Autodesk Inventor part; units mm, degrees
ref_plane "YZ Plane" through (0, 0, 0) normal (1, 0, 0) x (0, 1, 0)
ref_plane "XZ Plane" through (0, 0, 0) normal (0, 1, 0) x (-1, 0, 0)
ref_plane "XY Plane" through (0, 0, 0) normal (0, 0, 1) x (1, 0, 0)
sketch "Body" plane through (0, 0, 0) normal (0, 0, 1) x (1, 0, 0)
  line L0 (-13.716, -23.495) -> (13.716, -23.495)
  line L1 (13.716, -23.495) -> (13.716, 23.495)
  line L2 (13.716, 23.495) -> (-13.716, 23.495)
  line L3 (-13.716, 23.495) -> (-13.716, -23.495)
  line L4 (-13.716, -23.495) -> (13.716, 23.495) construction
  line L5 (13.716, -23.495) -> (-13.716, 23.495) construction
  point P0 (0, 0)
  dimension "d0" = 27.432
  dimension "d1" = 46.99
extrude "BodyFeature" add sketch "Body" along normal blind 22.606
chamfer "OutsideChamfersFeature" distance 6 angle 45 2 edges at (13.716, 23.495, 11.303) (-13.716, 23.495, 11.303)
sketch "Mount" plane through (0, 0, 22.606) normal (0, 0, 1) x (1, 0, 0)
  line L0 (-24.5, -29.5) -> (24.5, -29.5) construction
  line L1 (24.5, -29.5) -> (24.5, 29.5) construction
  line L2 (24.5, 29.5) -> (-24.5, 29.5) construction
  line L3 (-24.5, 29.5) -> (-24.5, -29.5) construction
  line L4 (-24.5, -29.5) -> (24.5, 29.5) construction
  line L5 (24.5, -29.5) -> (-24.5, 29.5) construction
  line L6 (-13.5, 29.5) -> (13.5, 29.5)
  line L7 (-13.5, 29.5) -> (-24.5, 0)
  line L8 (13.5, 29.5) -> (24.5, 0)
  line L9 (-33.6, 0) -> (33.6, 0) construction
  line L10 (-13.5, -29.5) -> (13.5, -29.5)
  line L11 (-13.5, -29.5) -> (-24.5, 0)
  line L12 (13.5, -29.5) -> (24.5, 0)
  point P0 (0, 0)
  point P1 (0, 29.5)
  dimension "d7" = 59
  dimension "d8" = 49
  dimension "d9" = 27
extrude "MountFeature" add sketch "Mount" along normal blind 2.32
fillet "MountFilletsFeature" radius 1 6 edges at (-13.5, 29.5, 23.766) (13.5, 29.5, 23.766) (-24.5, 0, 23.766) (24.5, 0, 23.766) (13.5, -29.5, 23.766) (-13.5, -29.5, 23.766)
sketch "MountHoles" plane through (0, 0, 24.926) normal (0, 0, 1) x (1, 0, 0)
  line L0 (-34.3, 0) -> (34.3, 0) construction
  circle A0 centre (-20, 0) radius 1.75
  line L1 (0, -41.3) -> (0, 41.3) construction
  circle A1 centre (20, 0) radius 1.75
  point P0 (0, 0)
  dimension "d13" = 3.5
  dimension "d14" = 40
extrude "MountHolesFeature" cut sketch "MountHoles" against normal blind 3.5
sketch "FrontPanel" plane through (0, 0, 24.926) normal (0, 0, 1) x (1, 0, 0)
  line L0 (-14.15, -27.7568) -> (14.15, -27.7568)
  line L1 (14.15, -27.7568) -> (14.15, 27.7568)
  line L2 (14.15, 27.7568) -> (-14.15, 27.7568)
  line L3 (-14.15, 27.7568) -> (-14.15, -27.7568)
  line L4 (-14.15, -27.7568) -> (14.15, 27.7568) construction
  line L5 (14.15, -27.7568) -> (-14.15, 27.7568) construction
  line L6 (24.3697, 0.3494) -> (13.7426, 28.8494) construction
  point P0 (0, 0)
  dimension "d17" = 28.3
extrude "FrontPanelFeature" add sketch "FrontPanel" along normal blind 0.5
fillet "FrontPanelFilletsFeature" radius 1 4 edges at (-14.15, -27.7568, 25.176) (14.15, -27.7568, 25.176) (-14.15, 27.7568, 25.176) (14.15, 27.7568, 25.176)
sketch "PowerReceptacle" plane through (0, 0, 25.426) normal (0, 0, 1) x (1, 0, 0)
  line L0 (0, -41.3) -> (0, 41.3) construction
  line L1 (-12.3, 22) -> (12.3, 22) construction
  line L2 (12.3, 22) -> (12.3, 5.8) construction
  line L3 (12.3, 5.8) -> (-12.3, 5.8) construction
  line L4 (-12.3, 5.8) -> (-12.3, 22) construction
  line L5 (-12.3, 22) -> (12.3, 5.8) construction
  line L6 (12.3, 22) -> (-12.3, 5.8) construction
  line L7 (12.8056, 29.5) -> (-12.8056, 29.5) construction
  line L8 (-7, 22) -> (7, 22)
  line L9 (-7, 22) -> (-12.3, 17.8)
  line L10 (-12.3, 17.8) -> (-12.3, 5.8)
  line L11 (7.716, 23.495) -> (-7.716, 23.495)
  line L12 (7, 22) -> (12.3, 17.8)
  line L13 (12.3, 17.8) -> (12.3, 5.8)
  line L14 (-12.3, 5.8) -> (12.3, 5.8)
  line L15 (14.15, 26.7568) -> (14.15, -26.7568)
  point P0 (0, 0)
  point P1 (0, 13.9)
  point P2 (0, 22)
  dimension "d22" = 24.6
  dimension "d23" = 16.2
  dimension "d24" = 7.5
  dimension "d25" = 14
  dimension "d26" = 12
extrude "PowerReceptacleFeature" cut sketch "PowerReceptacle" against normal blind 18.2
sketch "Switch" plane through (0, 0, 25.426) normal (0, 0, 1) x (1, 0, 0)
  line L0 (0, -41.3) -> (0, 41.3) construction
  line L1 (-12.3, -8.15) -> (12.3, -8.15)
  line L2 (12.3, -8.15) -> (12.3, -24)
  line L3 (12.3, -24) -> (-12.3, -24)
  line L4 (-12.3, -24) -> (-12.3, -8.15)
  line L5 (-12.3, -8.15) -> (12.3, -24) construction
  line L6 (12.3, -8.15) -> (-12.3, -24) construction
  line L7 (-12.8056, -29.5) -> (12.8056, -29.5)
  line L8 (-12.3, 5.8) -> (-12.3, 17.8)
  line L9 (12.3, 17.8) -> (12.3, 5.8)
  point P0 (0, 0)
  point P1 (0, -16.075)
  dimension "d29" = 5.5
  dimension "d30" = 15.85
extrude "SwitchFeature" add sketch "Switch" along normal blind 5.75
sketch "SwitchProfile" plane through (-12.3, -24, 25.426) normal (0, -1, 0) x (1, 0, 0)
  line L0 (24.6, 0) -> (0, 0)
  line L1 (24.6, 0) -> (24.6, 5.75)
  line L2 (0, 5.75) -> (24.6, 5.75)
  line L3 (0, 0) -> (0, 5.75)
  arc A0 (0, 0) -> (24.6, 5.75) centre (-4.9882, 76.8383) ccw
  point P0 (12.3, -25.426)
  dimension "d33" = 77
extrude "SwitchProfileFeature" cut sketch "SwitchProfile" against normal up to surface (15.85 mm away) contours L3 L2 A0
equation "\"d15\" = d13"
properties part number "AC-14-F16A"
The listing builds one solid part. Answer for the finished solid, in the listing's coordinates (mm). A direction names the side the tool comes from. Round coordinates to 2 decimals unless told otherwise and drop trailing zeros. Order: outer loops, then holes, each group sorted by start corner. A loop starts at its lowest first (then second) coordinate and runs counter-clockwise, first axis right, second up. Notation, with made-up numbers: (80, -0.75) -> (111, -0.75) arc R6 cw to (111, 8.25) -> close; hole circle Ø6 at (-3.5, 74.25). An arc over 180 degrees is marked (long way). Write each question's results on one line, items separated by ' | '. Start each with the question number.
Q1. Straight lines are drawn through the part: probe 1 along Y at (x, z) = (5.5, 7.5) (3 decimals); probe 2 along X at (y, z) = (-7, 13); probe 3 along Z at (x, y) = (10.5, 10.5). For each, find the intervals that lie inside material, in ascending order. Write a range as from..to.
Q2. The mould has two halves that part along X. Classify faces 6 (the cylindrical face through (-21.75, 0.08, 23.78)), 7 (the flat face through (18.98, 14.8, 23.75)), 8 (the flat face through (6, -24, 27)), 9 (the flat face through (0, 5.8, 16)): pulls with the +X half, pulls with the -X half, needs draft (parallel to the pull), parting line crosses it, or undercut.
Q3. Find section D-D (z = 4.5). Determine the outline of the cut face in (x, y) (3 decimals), then the cut area to 3 significant figures.
Q4. Find section B-B (z = 21.5). Determine the outline of the cut face in (x, y) (3 decimals).
Q5. Each of these flat-tipped pins is pushed along its axis until it touches: pin 1 (3 mm diameter, centred on y = -16, z = 26, fed in from -X); pin 2 (10 mm diameter, centred on x = -18.5, z = 12, fed in from +Y); pin 3 (6 mm diameter, centred on y = -7.5, z = 3.5, fed in from +X). Where does it stop, or does it pass through?
Q6. Find section C-C (y = 3.5). Determine the outline of the cut face in (x, z).
Q7. Which of the six approach directions +Z, -Z, +X, -X, +Y, -Y give full straight-line access (tool end or side, diameter ignored) to faces 1 (the flat face through (-13.716, -3, 11)), 2 (the flat face through (0, -23.495, 11)), 3 (the flat face through (0, 23.495, 11)), 4 (the flat face through (-9.61, 19.93, 16.45)), 5 (the flat face through (10.76, 20.45, 11.14))?
Q8. Find section A-A (x = 20). Determine the outline of the cut face in (y, z).
Worked answers:
1) probe 1: y = -23.495..5.8, 22..23.495 | probe 2: x = -13.72..13.72 | probe 3: z = 0..7.23
2) face 6: undercut | face 7: pulls with the +X half | face 8: needs draft | face 9: undercut
3) outline: (-13.716, -23.495) -> (13.716, -23.495) -> (13.716, 17.495) -> (7.716, 23.495) -> (-7.716, 23.495) -> (-13.716, 17.495) -> close | area: 1,250 mm2
4) outline: (-13.716, -23.495) -> (13.716, -23.495) -> (13.716, 17.495) -> (7.716, 23.495) -> (-7.716, 23.495) -> (-13.716, 17.495) -> close; hole (-12.3, 5.8) -> (12.3, 5.8) -> (12.3, 17.8) -> (7, 22) -> (-7, 22) -> (-12.3, 17.8) -> close
5) pin 1: stops at x = -18.92 | pin 2: stops at y = 17.71 | pin 3: stops at x = 13.72
6) outline: (-23.19, 22.61) -> (-13.72, 22.61) -> (-13.72, 0) -> (13.72, 0) -> (13.72, 22.61) -> (23.19, 22.61) -> (23.19, 24.93) -> (14.15, 24.93) -> (14.15, 25.43) -> (-14.15, 25.43) -> (-14.15, 24.93) -> (-23.19, 24.93) -> close
7) face 1: -Z, -X, +Y, -Y | face 2: -Z, +X, -X, -Y | face 3: -Z, +X, -X, +Y | face 4: +Z | face 5: -Z, +X, +Y
8) outline: (-12.07, 22.61) -> (-1.75, 22.61) -> (-1.75, 24.93) -> (-12.07, 24.93) -> close; (1.75, 22.61) -> (12.07, 22.61) -> (12.07, 24.93) -> (1.75, 24.93) -> close
